Part model, mm, in its own coordinate system. A direction names the side the tool comes from. Coordinates: 2 decimals unless noted, no trailing zeros. Write each loop counter-clockwise with the first axis right and the second up, starting at its lowest first coordinate (ties: lowest second). Pieces come first, ordered by that corner, then holes. Notation, with made-up numbers: (-34.75, 82) - (-30.75, 82) arc R22 ccw to (-30.75, 93) - close; hole circle Ø10 at (43.25, 62). An arc over 180 degrees is marked (long way). Use one line per item in the form item = value. Start each with the question number.
from build123d import *

# Parameters (mm, degrees)
SKETCH2_R           = 35
SKETCH2_R_2         = 5
BOSS_EXTRUDE1_DEPTH = 5
SKETCH3_R           = 20
SKETCH3_R_2         = 15
BOSS_EXTRUDE3_DEPTH = 15
SKETCH4_R           = 1.6
CUT_EXTRUDE1_DEPTH  = 59.940648113
CIRPATTERN1_COUNT   = 4


with BuildPart() as part:
    # Sketch2 → Boss-Extrude1 (new body)
    with BuildSketch(Plane.XY):
        Circle(SKETCH2_R)
        Circle(SKETCH2_R_2, mode=Mode.SUBTRACT)
    extrude(amount=BOSS_EXTRUDE1_DEPTH)

    # Sketch3 → Boss-Extrude3 (add)
    # profile 1 of 9: a face of its own
    with BuildSketch(Plane.XY.offset(5)):
        with BuildLine():
            ThreePointArc((-3, -19.773719933), (-5.547149112, -19.215335978), (-8, -18.33030278))
            Line((-8, -18.33030278), (-8, -34.073450075))
            ThreePointArc((-8, -34.073450075), (-5.514444475, -34.562854369), (-3, -34.871191548))
            Line((-3, -34.871191548), (-3, -19.773719933))
        make_face()
    # profile 2 of 9: a face of its own
    with BuildSketch(Plane.XY.offset(5)):
        with BuildLine():
            Line((8, -34.073450075), (8, -18.33030278))
            ThreePointArc((8, -18.33030278), (5.547149112, -19.215335978), (3, -19.773719933))
            Line((3, -19.773719933), (3, -34.871191548))
            ThreePointArc((3, -34.871191548), (5.514444475, -34.562854369), (8, -34.073450075))
        make_face()
    # profile 3 of 9: a face of its own
    with BuildSketch(Plane.XY.offset(5)):
        with BuildLine():
            Line((34.871191548, -3), (19.773719933, -3))
            ThreePointArc((19.773719933, -3), (19.215335978, -5.547149112), (18.33030278, -8))
            Line((18.33030278, -8), (34.073450075, -8))
            ThreePointArc((34.073450075, -8), (34.562854369, -5.514444475), (34.871191548, -3))
        make_face()
    # profile 4 of 9: a face of its own
    with BuildSketch(Plane.XY.offset(5)):
        with BuildLine():
            Line((34.073450075, 8), (18.33030278, 8))
            ThreePointArc((18.33030278, 8), (19.215335978, 5.547149112), (19.773719933, 3))
            Line((19.773719933, 3), (34.871191548, 3))
            ThreePointArc((34.871191548, 3), (34.562854369, 5.514444475), (34.073450075, 8))
        make_face()
    # profile 5 of 9: a face of its own
    with BuildSketch(Plane.XY.offset(5)):
        with BuildLine():
            Line((3, 34.871191548), (3, 19.773719933))
            ThreePointArc((3, 19.773719933), (5.547149112, 19.215335978), (8, 18.33030278))
            Line((8, 18.33030278), (8, 34.073450075))
            ThreePointArc((8, 34.073450075), (5.514444475, 34.562854369), (3, 34.871191548))
        make_face()
    # profile 6 of 9: a face of its own
    with BuildSketch(Plane.XY.offset(5)):
        with BuildLine():
            ThreePointArc((-8, 18.33030278), (-5.547149112, 19.215335978), (-3, 19.773719933))
            Line((-3, 19.773719933), (-3, 34.871191548))
            ThreePointArc((-3, 34.871191548), (-5.514444475, 34.562854369), (-8, 34.073450075))
            Line((-8, 34.073450075), (-8, 18.33030278))
        make_face()
    # profile 7 of 9: a face of its own
    with BuildSketch(Plane.XY.offset(5)):
        with BuildLine():
            ThreePointArc((-19.773719933, 3), (-19.215335978, 5.547149112), (-18.33030278, 8))
            Line((-18.33030278, 8), (-34.073450075, 8))
            ThreePointArc((-34.073450075, 8), (-34.562854369, 5.514444475), (-34.871191548, 3))
            Line((-34.871191548, 3), (-19.773719933, 3))
        make_face()
    # profile 8 of 9: a face of its own
    with BuildSketch(Plane.XY.offset(5)):
        with BuildLine():
            ThreePointArc((-18.33030278, -8), (-19.215335978, -5.547149112), (-19.773719933, -3))
            Line((-19.773719933, -3), (-34.871191548, -3))
            ThreePointArc((-34.871191548, -3), (-34.562854369, -5.514444475), (-34.073450075, -8))
            Line((-34.073450075, -8), (-18.33030278, -8))
        make_face()
    # profile 9 of 9: a face of its own
    with BuildSketch(Plane.XY.offset(5)):
        Circle(SKETCH3_R)
        Circle(SKETCH3_R_2, mode=Mode.SUBTRACT)
    extrude(amount=BOSS_EXTRUDE3_DEPTH)

    # Sketch4 → Cut-Extrude1 (cut, through all)
    with BuildSketch(Plane.ZY.offset(8)):
        with Locations((12.5, 26.596250524)):
            Circle(SKETCH4_R)
    cut_extrude1 = extrude(amount=-CUT_EXTRUDE1_DEPTH, mode=Mode.SUBTRACT)

    # CirPattern1: Cut-Extrude1 ×4 about axis
    cirpattern1_axis = Axis((0, 0, 20), (0, 0, -1))
    for i in range(1, CIRPATTERN1_COUNT):
        add(cut_extrude1.rotate(cirpattern1_axis, i * 360 / CIRPATTERN1_COUNT), mode=Mode.SUBTRACT)


solid = part.part
Q1. Pin check, flat tips, straight feed: P1, Ø3, axis at x = -25.5, y = 0.5, coming from the +Z side; P2, Ø12, axis at x = -10.5, z = 10, coming from the +Y side; P3, Ø7.5, axis at y = -24.5, z = 12.5, coming from the +X side. Stop position of each tip, or through.
Q2. Mould opens along Z. For faces 1 (the cylindrical face through (-5.46, -25.62, 11.23)), 2 (the cylindrical face through (25.62, 5.54, 11.23)), 3 (the flat face through (29, 3, 12)), 4 (the flat face through (0, 27, 5)) say: released by +Z, released by -Z, zero draft, split by the parting line, or undercut.
Q3. Slice it at A-A (y = 0). List the corners of the cut face in (x, z), plus the area to 3 significant figures.
Q4. Drill centre lines: probe 1 along X at (y, z) = (21.5, 9); probe 2 along Y at (x, z) = (-6.5, 12). Where is each one in solid material? Low to high.
Q5. Which spindle directions (+Z, -Z, +X, -X, +Y, -Y) get a long thin tool onto all of the face, cutting with end or side? Do faces 5 (the flat face through (3, 29, 12)), 6 (the flat face through (26.3, 8, 10.7)), 7 (the flat face through (27, 0, 5)), 8 (the flat face through (-18, 18, 5)). Say none if no direction does.
Q6. Slice it at D-D (z = 12.5). Count the separate pieces of the cut face and the enclosed holes in it, plus the area to 3 significant figures.
Solution:
q1.P1 = 5
q1.P2 = 34.71
q1.P3 = 8
q2.face_1 = undercut
q2.face_2 = undercut
q2.face_3 = zero draft
q2.face_4 = released by +Z
q3.outline = (-35, 0) - (-5, 0) - (-5, 5) - (-15, 5) - (-15, 20) - (-20, 20) - (-20, 5) - (-35, 5) - close; (5, 0) - (35, 0) - (35, 5) - (20, 5) - (20, 20) - (15, 20) - (15, 5) - (5, 5) - close
q3.area = 450 mm2
q4.probe_1 = -8 to -3, 3 to 8
q4.probe_2 = -34.39 to -28.12, -25.08 to -13.52, 13.52 to 25.08, 28.12 to 34.39
q5.face_5 = +Z, +Y
q5.face_6 = +Z, +X, +Y
q5.face_7 = +Z, +X
q5.face_8 = +Z, -X, +Y
q6.separate_pieces = 9
q6.enclosed_holes = 1
q6.area = 1,040 mm2
